from build123d import *

# Parameters (mm, degrees)
F0_R      = 22.5
F1_DEPTH  = 50
F2_W      = 46
F2_H      = 50
F2_R      = 22.5
F3_DEPTH  = 70
F4_R      = 22.5
F5_DEPTH  = 50
F6_R      = 17.5
F7_DEPTH  = 20
F8_R      = 17.5
F9_DEPTH  = 20
F10_W     = 28
F10_H     = 38
F11_DEPTH = 30.5
F12_W     = 28
F12_H     = 38
F13_DEPTH = 30.5
F15_R     = 2.5
F16_DEPTH = 50
F14_R     = 4.5
F17_DEPTH = 11
F18_W     = 6
F18_H     = 0.9020372182
F19_DEPTH = 11
F20_W     = 6
F20_H     = 1
F21_DEPTH = 11
F20_W_2   = 1
F20_H_2   = 5
F22_DEPTH = 10
F18_W_2   = 0.9020372182
F18_H_2   = 5
F23_DEPTH = 10


# Not quite as in the source:
# - a feature names something its author has since deleted; it is built from what else it names


with BuildPart() as f1:
    # F0 (on Front) → F1 (new body)
    with BuildSketch(Plane.XZ):
        Circle(F0_R)
    extrude(amount=F1_DEPTH)

    # F2 (on face) → F3 (join)
    with BuildSketch(Plane.XZ.offset(50)):
        with Locations((0, 2)):
            Rectangle(F2_W, F2_H)
        Circle(F2_R, mode=Mode.SUBTRACT)
        Circle(F2_R)
    extrude(amount=F3_DEPTH)

    # F4 (on face) → F5 (join)
    with BuildSketch(Plane.XZ.offset(120)):
        Circle(F4_R)
    extrude(amount=F5_DEPTH)

    # F6 (on face) → F7 (join)
    with BuildSketch(Plane.XZ.offset(170)):
        Circle(F6_R)
    extrude(amount=F7_DEPTH)

    # F8 (on face) → F9 (join)
    with BuildSketch(Plane(origin=(0, 0, 0), x_dir=(-1, 0, 0), z_dir=(0, 1, 0))):
        Circle(F8_R)
    extrude(amount=F9_DEPTH)

    # F10 (on Top) → F11 (join)
    with BuildSketch(Plane.XY):
        with Locations((0, -29)):
            Rectangle(F10_W, F10_H)
    extrude(amount=F11_DEPTH)

    # F12 (on Top) → F13 (join)
    with BuildSketch(Plane.XY):
        with Locations((0, -141)):
            Rectangle(F12_W, F12_H)
    extrude(amount=F13_DEPTH)

    # F15 (on face) → F16 (cut)
    with BuildSketch(Plane.XY.offset(27)):
        with Locations((-15.5, -64.5)):
            Circle(F15_R)
        with Locations((-15.5, -105.5)):
            Circle(F15_R)
        with Locations((15.5, -105.5)):
            Circle(F15_R)
        with Locations((15.5, -64.5)):
            Circle(F15_R)
    extrude(amount=-F16_DEPTH, mode=Mode.SUBTRACT)

    # F14 (on face) → F17 (cut)
    with BuildSketch(Plane.XY.offset(27)):
        with Locations((-15.5, -64.5)):
            Circle(F14_R)
        with Locations((15.5, -64.5)):
            Circle(F14_R)
        with Locations((15.5, -105.5)):
            Circle(F14_R)
        with Locations((-15.5, -105.5)):
            Circle(F14_R)
    extrude(amount=-F17_DEPTH, mode=Mode.SUBTRACT)

    # F18 (on face) → F19 (join)
    with BuildSketch(Plane.XY.offset(30.5)):
        with Locations((0, -42.164042592)):
            Rectangle(F18_W, F18_H)
    extrude(amount=F19_DEPTH)

    # F20 (on face) → F21 (join)
    with BuildSketch(Plane.XY.offset(30.5)):
        with Locations((0, -128.5)):
            Rectangle(F20_W, F20_H)
    extrude(amount=F21_DEPTH)

    # F20 (on face) → F22 (join)
    with BuildSketch(Plane.XY.offset(30.5)):
        with Locations((9.5, -136.5)):
            Rectangle(F20_W_2, F20_H_2)
        with Locations((0, -128.5)):
            Rectangle(F20_W, F20_H)
        with Locations((-9.5, -136.5)):
            Rectangle(F20_W_2, F20_H_2)
    extrude(amount=F22_DEPTH)

    # F18 (on face) → F23 (join)
    with BuildSketch(Plane.XY.offset(30.5)):
        with Locations((-9.5489813909, -32.5)):
            Rectangle(F18_W_2, F18_H_2)
        with Locations((9.5489813909, -32.5)):
            Rectangle(F18_W_2, F18_H_2)
        with Locations((0, -42.164042592)):
            Rectangle(F18_W, F18_H)
    extrude(amount=F23_DEPTH)


solid = f1.part
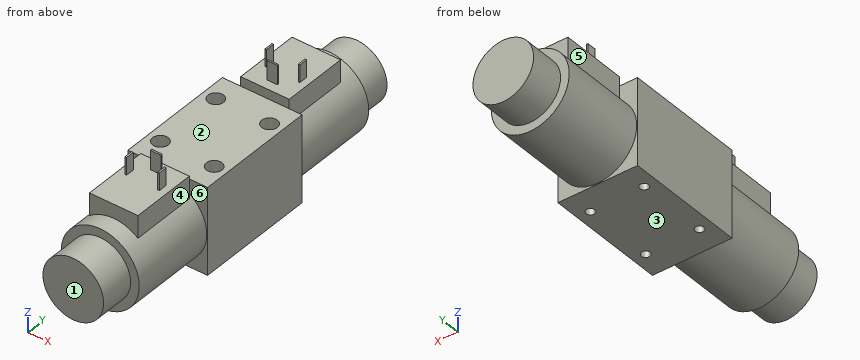
Source: CAD feature listing. Evaluate the final solid. Frame: model axes, mm. Face numbers are marked on the shaded views. A direction names the side the tool comes from. Give positions to 0.01 mm unless a question says otherwise; leave off trailing zeros. Write each loop counter-clockwise with the first axis right and the second up, starting at its lowest first coordinate (ties: lowest second). Pieces come first, ordered by that corner, then holes. Notation, with made-up numbers: M 63.25,-26.75 L 111.25,-26.75 A31 ccw 111.25,-2.75 Z; hole C 86,69.25 d11. An arc over 180 degrees is marked long. Answer as a JSON object with one key per item and string values.
Q1. Ray query, line 1 along X through (y, z) = (-64, 23); line 2 along Y through (x, z) = (15.5, -9); line 3 along Y through (x, z) = (15, 23). Return the intervals inside material, ascending.
Geometry check:
{"line 1": "x = -23 to -19.97, -11.03 to 11.03, 19.97 to 23", "line 2": "y = -170 to -108, -103 to -67, -62 to 0", "line 3": "y = -120 to -109.97, -101.03 to -68.97, -60.03 to -50"}
Q2. Cut plane A-A, the plane z = 35.5. Return the cut outline in (x, y).
Geometry check:
{"outline": "M -10,-139 L -9,-139 L -9,-134 L -10,-134 Z; M -10,-35 L -9.1,-35 L -9.1,-30 L -10,-30 Z; M -3,-129 L 3,-129 L 3,-128 L -3,-128 Z; M -3,-42.62 L 3,-42.62 L 3,-41.71 L -3,-41.71 Z; M 9,-139 L 10,-139 L 10,-134 L 9,-134 Z; M 9.1,-35 L 10,-35 L 10,-30 L 9.1,-30 Z"}
Q3. Mould query, pull axis Y, two halves, no side actions, for the marked faces 1, 2 and 3. Classes: +Y half, -Y half, draft (parallel to the pull), parting line (faces both ways), or undercut.
Geometry check:
{"face 1": "-Y half", "face 2": "undercut", "face 3": "draft"}
Q4. Cut plane D-D, the plane x = 5.5. Return the cut outline in (y, z).
Geometry check:
{"outline": "M -190,-16.61 L -170,-16.61 L -170,-21.82 L -120,-21.82 L -120,-23 L -50,-23 L -50,-21.82 L 0,-21.82 L 0,-16.61 L 20,-16.61 L 20,16.61 L 0,16.61 L 0,21.82 L -10,21.82 L -10,30.5 L -48,30.5 L -48,21.82 L -50,21.82 L -50,27 L -120,27 L -120,21.82 L -122,21.82 L -122,30.5 L -160,30.5 L -160,21.82 L -170,21.82 L -170,16.61 L -190,16.61 Z"}
Q5. Cut plane C-C, the plane z = 0. Return the cut outline in (x, y).
Geometry check:
{"outline": "M -23,-120 L -22.5,-120 L -22.5,-170 L -17.5,-170 L -17.5,-190 L 17.5,-190 L 17.5,-170 L 22.5,-170 L 22.5,-120 L 23,-120 L 23,-50 L 22.5,-50 L 22.5,0 L 17.5,0 L 17.5,20 L -17.5,20 L -17.5,0 L -22.5,0 L -22.5,-50 L -23,-50 Z; hole C -15.5,-105.5 d5; hole C -15.5,-64.5 d5; hole C 15.5,-105.5 d5; hole C 15.5,-64.5 d5"}
Q6. Cut plane B-B, the plane y = -64.5. Return the cut outline in (x, z).
Geometry check:
{"outline": "M -23,-23 L -18,-23 L -18,16 L -20,16 L -20,27 L -23,27 Z; M -13,-23 L 13,-23 L 13,16 L 11,16 L 11,27 L -11,27 L -11,16 L -13,16 Z; M 18,-23 L 23,-23 L 23,27 L 20,27 L 20,16 L 18,16 Z"}
Q7. Access query for the marked faces 4, 5 and 6. Directions: +Z, -Z, +X, -X, +Y, -Y. A direction counts if a zero-diameter tool reaches every point of the face in a straight line with its end or side. Return the directions, or none.
Geometry check:
{"face 4": "+Z, +X, -Y", "face 5": "+Z, -X, +Y", "face 6": "none"}
Q8. Contact query for flat-ended pins moving along their axis: P1, Ø10, axis at y = -19, z = 20, coming from the -X side; P2, Ø6, axis at x = -14.5, y = -48, coming from the -Z side; P3, Ø0.8, axis at x = 9.5, y = -137.5, coming from the +Z side; P4, Ø1.5, axis at y = -33, z = 37, coming from the -X side. Output: stop coordinate, or through.
Geometry check:
{"P1": "stops at x = -16.77", "P2": "stops at z = -23", "P3": "stops at z = 40.5", "P4": "stops at x = -10"}
